For this review, use the dimensioned drawing (mm, ordinates from the lowest corner) and the shaded views. A direction names the side the tool comes from. Coordinates: 2 decimals unless noted, no trailing zeros. Order: outer loops, then holes, each group sorted by start corner. A loop starts at its lowest first (then second) coordinate and runs counter-clockwise, first axis right, second up. Notation, with made-up numbers: M 76,56.5 L 98,56.5 A35 ccw 98,92.5 Z; hole C 18.5,33.5 d5. An arc over 180 degrees is marked long. Answer in a Markdown table with one row per item.
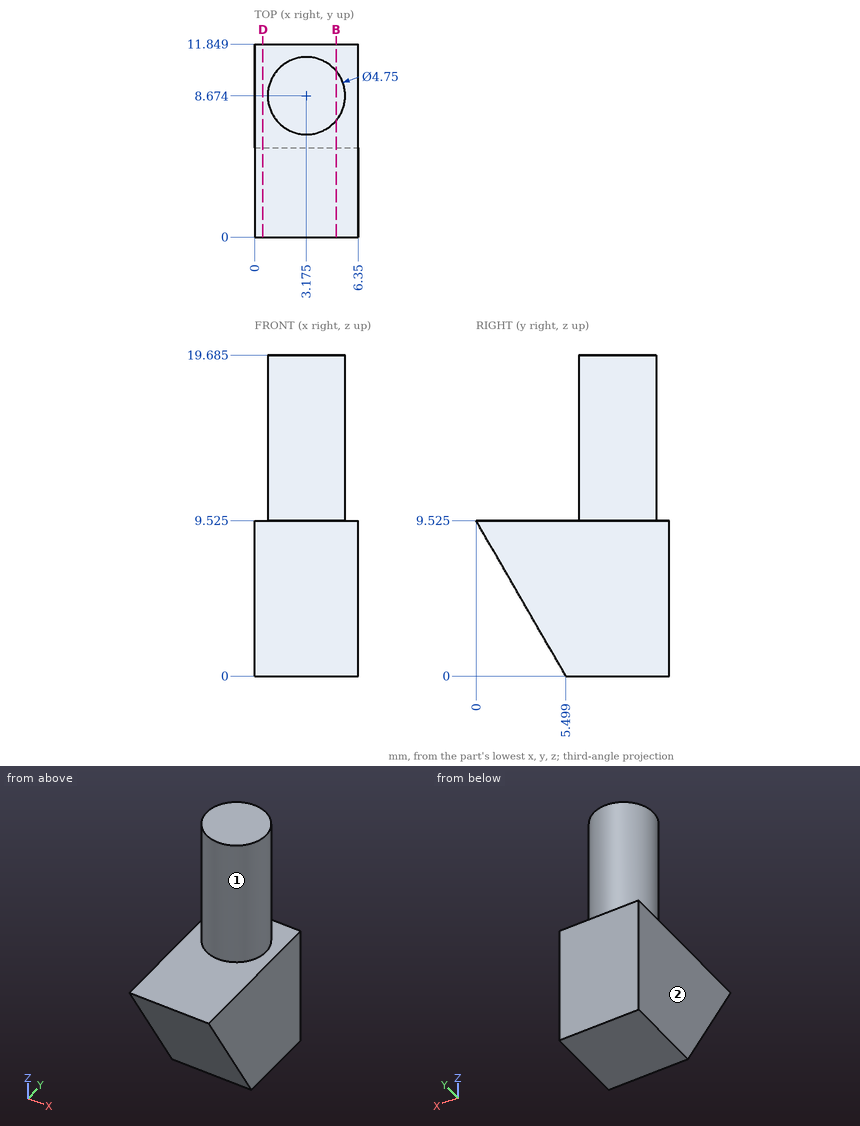
(1) Insertion check: pin 1 Ø2 at (x, z) = (3.5, 6.5) entering from -Y. The pin has a flat end and moves straight along its axis. Give the tip position at first contact, or say it passes through.
Return value:
| item | result |
|---|---|
| pin 1 | stops at y = 1.17 |
(2) For line 1 along X through (y, z) = (8.75, 18.75); line 2 along Y through (x, z) = (3.25, 11.25); line 3 along Z through (x, y) = (5.25, 11.5) (1 decimal), list the stretches that pass through material, from the lowest coordinate up. Write a range as from..to.
Return value:
| item | result |
|---|---|
| line 1 | x = 0.8..5.55 |
| line 2 | y = 6.3..11.05 |
| line 3 | z = 0..9.5 |
(3) Add section D-D, the plane x = 0.5. Give the boundary of the cut face in (y, z) (1 decimal).
Return value:
| item | result |
|---|---|
| outline | M 0,9.5 L 5.5,0 L 11.8,0 L 11.8,9.5 Z |
(4) For the marked faces 1 and 2, list the 3-axis set-ups (+Z, -Z, +X, -X, +Y, -Y) from which the entire face can be reached by the end or side of a thin tool; tool diameter is ignored.
Return value:
| item | result |
|---|---|
| face 1 | +Z |
| face 2 | +Z, -Z, -X, +Y, -Y |
(5) Add section B-B, the plane x = 5. Give the boundary of the cut face in (y, z) (1 decimal).
Return value:
| item | result |
|---|---|
| outline | M 0,9.5 L 5.5,0 L 11.8,0 L 11.8,9.5 L 10.2,9.5 L 10.2,19.7 L 7.2,19.7 L 7.2,9.5 Z |
